```python
from build123d import *

# Parameters (mm, degrees)
SKETCH1_R           = 41.91
BOSS_EXTRUDE1_DEPTH = 12.7
SKETCH2_R           = 13.97
CUT_EXTRUDE1_DEPTH  = 12.7
SKETCH2_3_R         = 26.67
SKETCH2_3_R_2       = 13.97
CUT_EXTRUDE2_DEPTH  = 12.7
SCALE1_SCALE        = 2
SCALE2_SCALE        = 0.5
SKETCH3_R           = 2.54
CUT_EXTRUDE3_DEPTH  = 12.7
CIRPATTERN1_COUNT   = 4


with BuildPart() as part:
    # Sketch1 → Boss-Extrude1 (new body)
    with BuildSketch(Plane(origin=(0, 0, 0), x_dir=(1, 0, 0), z_dir=(0, 1, 0))):
        with Locations(Location((0, 0, 0), (0, 0, 270))):
            Circle(SKETCH1_R)
    extrude(amount=BOSS_EXTRUDE1_DEPTH)

    # Sketch2 → Cut-Extrude1 (cut)
    with BuildSketch(Plane(origin=(0, 12.7, 0), x_dir=(1, 0, 0), z_dir=(0, 1, 0))):
        with Locations(Location((0, 0, 0), (0, 0, 270))):
            Circle(SKETCH2_R)
    extrude(amount=-CUT_EXTRUDE1_DEPTH, mode=Mode.SUBTRACT)

    # Sketch2<3> → Cut-Extrude2 (cut)
    with BuildSketch(Plane(origin=(0, 12.7, 0), x_dir=(1, 0, 0), z_dir=(0, 1, 0))):
        with Locations(Location((0, 0, 0), (0, 0, 270))):
            Circle(SKETCH2_3_R)
        Circle(SKETCH2_3_R_2, mode=Mode.SUBTRACT)
    extrude(amount=-CUT_EXTRUDE2_DEPTH, mode=Mode.SUBTRACT)


with BuildPart() as part_1:
    # Scale1: scaled about (0, 6.35, 0)
    add(part.part.scale(SCALE1_SCALE).moved(Location((0, -6.35, 0))))


with BuildPart() as part_2:
    # Scale2: scaled about (0, 6.35, 0)
    add(part_1.part.scale(SCALE2_SCALE).moved(Location((0, 3.175, 0))))

    # Sketch3 → Cut-Extrude3 (cut)
    with BuildSketch(Plane(origin=(0, 12.7, 0), x_dir=(1, 0, 0), z_dir=(0, 1, 0))):
        with Locations(Location((0, 38.1, 0), (0, 0, 270))):
            Circle(SKETCH3_R)
    cut_extrude3 = extrude(amount=-CUT_EXTRUDE3_DEPTH, mode=Mode.SUBTRACT)

    # CirPattern1: Cut-Extrude3 ×4 about axis
    cirpattern1_axis = Axis((0, 0, 0), (0, 1, 0))
    for i in range(1, CIRPATTERN1_COUNT):
        add(cut_extrude3.rotate(cirpattern1_axis, i * 360 / CIRPATTERN1_COUNT), mode=Mode.SUBTRACT)


solid = part_2.part
```
Here's how the part is built. I have some questions about the finished solid (model axes, mm). Round coordinates to 2 decimals unless told otherwise and drop trailing zeros. Write each loop counter-clockwise with the first axis right and the second up, starting at its lowest first coordinate (ties: lowest second). Pieces come first, ordered by that corner, then holes.
Q1. If we section it at C-C on y = 4: Write out the boundary of the cut face in (x, z).
Q2. If we section it at A-A on z = 0: Write out the boundary of the cut face in (x, y), plus the area to 3 significant figures.
Q3. If we mould it in two halves opening along Z, with no side actions, what happens to faces 1 (the cylindrical face through (-40.638, 6.439, -0.112)), 2 (the cylindrical face through (35.34, 6.26, 22.53)), 3 (the cylindrical face through (26.443, 6.439, -3.472)), 4 (the flat face through (-27, 0, -1))? For each: +Z half, -Z half, draft (parallel to the pull), parting line (faces both ways), or undercut.
Q4. If we section it at D-D on x = 10: Write out the boundary of the cut face in (y, z).
Q5. Please list where these lines run through material, in increasing order: probe 1 along Z at (x, y) = (3.5, 10.75); probe 2 along Z at (x, y) = (-38.1, 8.75).
Q6. If we section it at B-B on x = 0: Write out the boundary of the cut face in (y, z), plus the area to 3 significant figures.
Q7. Will these pins go through, and if not, where does the flat tip stop? P1, Ø5, axis at x = 18.5, y = 4, coming from the -Z side; P2, Ø1, axis at x = -21, y = 3.5, coming from the +Z side; P3, Ø6, axis at y = 7.5, z = -12, coming from the +X side.
Answer below:
1. outline: circle Ø83.82 at (0, 0); hole circle Ø5.08 at (-38.1, 0); hole circle Ø53.34 at (0, 0); hole circle Ø5.08 at (0, -38.1); hole circle Ø5.08 at (0, 38.1); hole circle Ø5.08 at (38.1, 0)
2. outline: (-41.91, 0) - (-40.64, 0) - (-40.64, 12.7) - (-41.91, 12.7) - close; (-35.56, 0) - (-26.67, 0) - (-26.67, 12.7) - (-35.56, 12.7) - close; (26.67, 0) - (35.56, 0) - (35.56, 12.7) - (26.67, 12.7) - close; (40.64, 0) - (41.91, 0) - (41.91, 12.7) - (40.64, 12.7) - close
2. area: 258 mm2
3. face 1: undercut
3. face 2: parting line
3. face 3: undercut
3. face 4: draft
4. outline: (0, -40.7) - (12.7, -40.7) - (12.7, -24.72) - (0, -24.72) - close; (0, 24.72) - (12.7, 24.72) - (12.7, 40.7) - (0, 40.7) - close
5. probe 1: z = -41.76 to -26.44, 26.44 to 41.76
5. probe 2: z = -17.46 to -2.54, 2.54 to 17.46
6. outline: (0, -41.91) - (12.7, -41.91) - (12.7, -40.64) - (0, -40.64) - close; (0, -35.56) - (12.7, -35.56) - (12.7, -26.67) - (0, -26.67) - close; (0, 26.67) - (12.7, 26.67) - (12.7, 35.56) - (0, 35.56) - close; (0, 40.64) - (12.7, 40.64) - (12.7, 41.91) - (0, 41.91) - close
6. area: 258 mm2
7. P1: stops at z = -38.74
7. P2: stops at z = 36.55
7. P3: stops at x = 40.93
